```python
from build123d import *

# Parameters (mm, degrees)
SKETCH1_W               = 60
SKETCH1_H               = 6.25
BOSS_EXTRUDE1_DEPTH     = 30
CUT_EXTRUDE1_DEPTH      = 68.372564891
CUT_EXTRUDE1_DEPTH_BACK = 45
SKETCH4_R               = 2.5
SKETCH4_W               = 15.6
SKETCH4_H               = 10.5
CUT_EXTRUDE2_DEPTH      = 4
CUT_EXTRUDE3_DEPTH      = 3.9


with BuildPart() as part:
    # Sketch1 → Boss-Extrude1 (new body)
    with BuildSketch(Plane(origin=(0, 0, 0), x_dir=(0, 0, -1), z_dir=(1, 0, 0))):
        with Locations((30, 3.125)):
            Rectangle(SKETCH1_W, SKETCH1_H)
    extrude(amount=BOSS_EXTRUDE1_DEPTH)

    # Sketch2 → Cut-Extrude1 (cut, two sides: drawn at the far end of the back side and taken through both)
    with BuildSketch(Plane.XY.offset(-CUT_EXTRUDE1_DEPTH_BACK)):
        with BuildLine():
            Line((5, 6.25), (25, 6.25))
            ThreePointArc((25, 6.25), (15, 2), (5, 6.25))
        make_face()
    extrude(amount=CUT_EXTRUDE1_DEPTH + CUT_EXTRUDE1_DEPTH_BACK, mode=Mode.SUBTRACT)

    # Sketch4 → Cut-Extrude2 (cut)
    with BuildSketch(Plane.XZ):
        with Locations(Location((15, -15.87, 0), (0, 0, 270))):
            Circle(SKETCH4_R)
        with Locations(Location((15, -22.52, 0), (0, 0, 270))):
            Circle(SKETCH4_R)
        with Locations(Location((15, -30.15, 0), (0, 0, 270))):
            Circle(SKETCH4_R)
        with Locations((15, -50.85)):
            Rectangle(SKETCH4_W, SKETCH4_H)
    extrude(amount=-CUT_EXTRUDE2_DEPTH, mode=Mode.SUBTRACT)

    # Sketch5 → Cut-Extrude3 (cut)
    with BuildSketch(Plane(origin=(0, 0, -60), x_dir=(-1, 0, 0), z_dir=(0, 0, -1))):
        Polygon((-10, 1.25), (-20, 1.25), (-18.5, 2.75), (-20, 4.25), (-10, 4.25), align=None)
    extrude(amount=-CUT_EXTRUDE3_DEPTH, mode=Mode.SUBTRACT)


solid = part.part
```
For this review, take the finished solid that the model builds, in its own axes (mm). A direction names the side the tool comes from. Coordinates: 2 decimals unless noted, no trailing zeros. Write each loop counter-clockwise with the first axis right and the second up, starting at its lowest first coordinate (ties: lowest second). Pieces come first, ordered by that corner, then holes. Notation, with made-up numbers: (-13, -12.75) - (19, -12.75) arc R10 ccw to (19, 0.25) - close; hole circle Ø9 at (-37.75, 62.25). An arc over 180 degrees is marked (long way). Answer in a Markdown table with one row per item. Add a question column.
Q1. Draft analysis for pull direction X (two halves, no side actions). For faces 1 (the flat face through (7.2, 2, -51)), 2 (the flat face through (0, 3, -30)), 3 (the flat face through (30, 3, -30)), 4 (the flat face through (14.8, 4.5, -60)), state which applies: +X half, -X half, draft (parallel to the pull), parting line (faces both ways), or undercut.
Q2. We need section A-A, the plane z = -15.87. State the section outline as (x, y) points, and give its area (3 significant figures).
Q3. We need section B-B, the plane x = 15. State the section outline as (y, z) points.
Q4. For P1, Ø1.3, axis at x = 13.5, y = 4.5, coming from the +Z side; P2, Ø3, axis at x = 12, z = -22, coming from the +Y side; P3, Ø1, axis at x = 19, z = -48.5, coming from the -Y side, all flat-tipped, find the tip position at first contact; note any pin that passes through.
Q5. Tool access review of faces 5 (the flat face through (15, 5, -45)), 6 (the flat face through (10, 3, -58)), 7 (the flat face through (4.8, 6.25, -36.2)), 8 (the flat face through (15, 2, -45.6)), 9 (the cylindrical face through (17.48, 1.1, -29.82)): name each direction out of +Z, -Z, +X, -X, +Y, -Y from which nothing blocks a thin tool from reaching the whole face with its end or side.
Q6. We need section C-C, the plane x = 11. State the section outline as (y, z) points.
Q7. We need section D-D, the plane z = -31.5. State the section outline as (x, y) points, and give its area (3 significant figures).
Q8. For probe 1 along Z at (x, y) = (15, 1.8); probe 2 along X at (y, z) = (0.9, -22.52); probe 3 along Z at (x, y) = (22.25, 3.75), list the stretches that pass through material, from the lowest coordinate up.
Answer list:
| question | item | result |
|---|---|---|
| 1 | face 1 | undercut |
| 1 | face 2 | -X half |
| 1 | face 3 | +X half |
| 1 | face 4 | draft |
| 2 | outline | (0, 0) - (12.5, 0) - (12.5, 2.23) arc R13.89 cw to (5, 6.25) - (0, 6.25) - close; (17.5, 0) - (30, 0) - (30, 6.25) - (25, 6.25) arc R13.89 cw to (17.5, 2.23) - close |
| 2 | area | 118 mm2 |
| 3 | outline | (0, -60) - (1.25, -60) - (1.25, -56.1) - (0, -56.1) - close; (0, -45.6) - (4, -45.6) - (4, -56.1) - (4.25, -56.1) - (4.25, -60) - (6.25, -60) - (6.25, -45) - (2, -45) - (2, -32.65) - (0, -32.65) - close; (0, -27.65) - (2, -27.65) - (2, -25.02) - (0, -25.02) - close; (0, -20.02) - (2, -20.02) - (2, -18.37) - (0, -18.37) - close; (0, -13.37) - (2, -13.37) - (2, 0) - (0, 0) - close |
| 4 | P1 | stops at z = -45 |
| 4 | P2 | stops at y = 2.75 |
| 4 | P3 | stops at y = 4 |
| 5 | face 5 | +Z, +Y |
| 5 | face 6 | -Z |
| 5 | face 7 | +Z, -Z, +X, -X, +Y |
| 5 | face 8 | -Y |
| 5 | face 9 | +Y, -Y |
| 6 | outline | (0, -60) - (1.25, -60) - (1.25, -56.1) - (0, -56.1) - close; (0, -45.6) - (4, -45.6) - (4, -56.1) - (4.25, -56.1) - (4.25, -60) - (6.25, -60) - (6.25, -45) - (2.59, -45) - (2.59, 0) - (0, 0) - close |
| 7 | outline | (0, 0) - (12.9, 0) - (12.9, 2.16) arc R13.89 cw to (5, 6.25) - (0, 6.25) - close; (17.1, 0) - (30, 0) - (30, 6.25) - (25, 6.25) arc R13.89 cw to (17.1, 2.16) - close |
| 7 | area | 120 mm2 |
| 8 | probe 1 | z = -45.6 to -32.65, -27.65 to -25.02, -20.02 to -18.37, -13.37 to 0 |
| 8 | probe 2 | x = 0 to 12.5, 17.5 to 30 |
| 8 | probe 3 | z = -60 to -56.1, -45.6 to 0 |
